Can you work these out from the drawing? Everything is in mm from the part's minimum corner. Round coordinates to 2 decimals unless told otherwise and drop trailing zeros. Write each loop counter-clockwise with the first axis right and the second up, starting at its lowest first coordinate (ties: lowest second). Pieces come first, ordered by that corner, then holes. Notation, with made-up numbers: M 40,72 L 54,72 A22 cw 54,78 Z; hole C 40,-31.5 d8. An arc over 180 degrees is marked long. Answer in a Markdown table with one row per item. Add a question column.
(1) Suppose I cut it at B-B, the plane x = 8. Write out the boundary of the cut face in (y, z).
(2) I'm going to push flat-ended pins straight in: pin 1 (1.5 mm diameter, centred on x = 14, z = 3.5, fed in from -Y) (3 decimals); pin 2 (2 mm diameter, centred on y = 7, z = 6, fed in from +X); pin 3 (1.5 mm diameter, centred on x = 7.5, z = 2.5, fed in from +Y). Where does each tip first touch, or does it pass through?
(3) If we mould it in two halves opening along Z, with no side actions, what happens to the marked faces 1, 2 and 3? For each: released by +Z, released by -Z, zero draft, split by the parting line, or undercut.
(4) If I drill on probe 1 along Y at (x, z) = (8, 6.7); probe 2 along Z at (x, y) = (14, 0.25); probe 3 along Z at (x, y) = (11, 2), over which ranges is the centre line in solid material (lowest first)?
(5) Suppose I cut it at D-D, the plane x = 2.25. Write out the boundary of the cut face in (y, z) (1 decimal).
(6) Suppose I cut it at A-A, the plane z = 4. Write out the boundary of the cut face in (x, y) (1 decimal).
(7) Suppose I cut it at C-C, the plane y = 7.5. Write out the boundary of the cut face in (x, z).
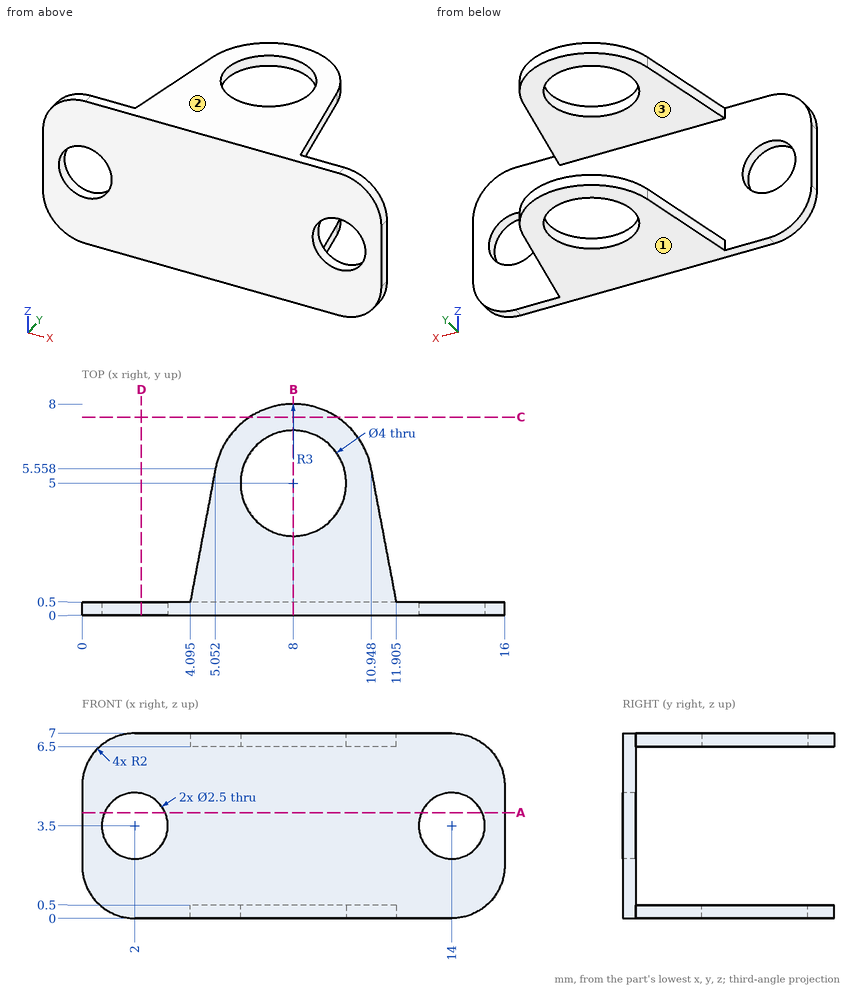
Calculated:
| question | item | result |
|---|---|---|
| 1 | outline | M 0,0 L 3,0 L 3,0.5 L 0.5,0.5 L 0.5,6.5 L 3,6.5 L 3,7 L 0,7 Z; M 7,0 L 8,0 L 8,0.5 L 7,0.5 Z; M 7,6.5 L 8,6.5 L 8,7 L 7,7 Z |
| 2 | pin 1 | through |
| 2 | pin 2 | x = 10.78 |
| 2 | pin 3 | y = 0.5 |
| 3 | face 1 | released by -Z |
| 3 | face 2 | released by +Z |
| 3 | face 3 | undercut |
| 4 | probe 1 | 0 to 3, 7 to 8 |
| 4 | probe 2 | 0 to 2.25, 4.75 to 7 |
| 4 | probe 3 | 0 to 0.5, 6.5 to 7 |
| 5 | outline | M 0,0 L 0.5,0 L 0.5,2.3 L 0,2.3 Z; M 0,4.7 L 0.5,4.7 L 0.5,7 L 0,7 Z |
| 6 | outline | M 0,0 L 0.9,0 L 0.9,0.5 L 0,0.5 Z; M 3.1,0 L 12.9,0 L 12.9,0.5 L 3.1,0.5 Z; M 15.1,0 L 16,0 L 16,0.5 L 15.1,0.5 Z |
| 7 | outline | M 6.34,0 L 9.66,0 L 9.66,0.5 L 6.34,0.5 Z; M 6.34,6.5 L 9.66,6.5 L 9.66,7 L 6.34,7 Z |
